Source: three-view drawing plus pictorial views. Frame: mm from the lowest corner of the part. Coordinates: 2 decimals unless noted, no trailing zeros. Order: outer loops, then holes, each group sorted by start corner. A loop starts at its lowest first (then second) coordinate and runs counter-clockwise, first axis right, second up. Notation, with made-up numbers: M -28,17 L 12,17 A24 cw 12,33 Z; hole C 38,-19.5 d11. An arc over 180 degrees is marked long. Use CSV: the item, a comma, the result in double quotes. Start each with the question number.
Q1. Section query B-B, the plane y = 7.25. Output: boundary loops of the cut face in (x, z), and give its area (3 significant figures).
Q2. Section query C-C, the plane z = 64. Output: boundary loops of the cut face in (x, y), and give its area (3 significant figures).
Q3. First-contact query: P1, Ø2.5, axis at y = 8, z = 28, coming from the +X side; P2, Ø3, axis at x = 1.5, y = 4, coming from the -Z side; P3, Ø1, axis at x = 2.5, z = 42, coming from the +Y side. Flat tips, straight axial feed; report the tip coordinate or a pass-through.
Q4. Section query D-D, the plane x = 4. Output: boundary loops of the cut face in (y, z), and give its area (3 significant figures).
Q5. Ray query, probe 1 along X at (y, z) = (2, 89.5); probe 2 along X at (y, z) = (4.75, 79); probe 3 along Z at (x, y) = (5.75, 1). Return the intervals inside material, ascending.
Q6. Section query A-A, the plane z = 8. Output: boundary loops of the cut face in (x, y).
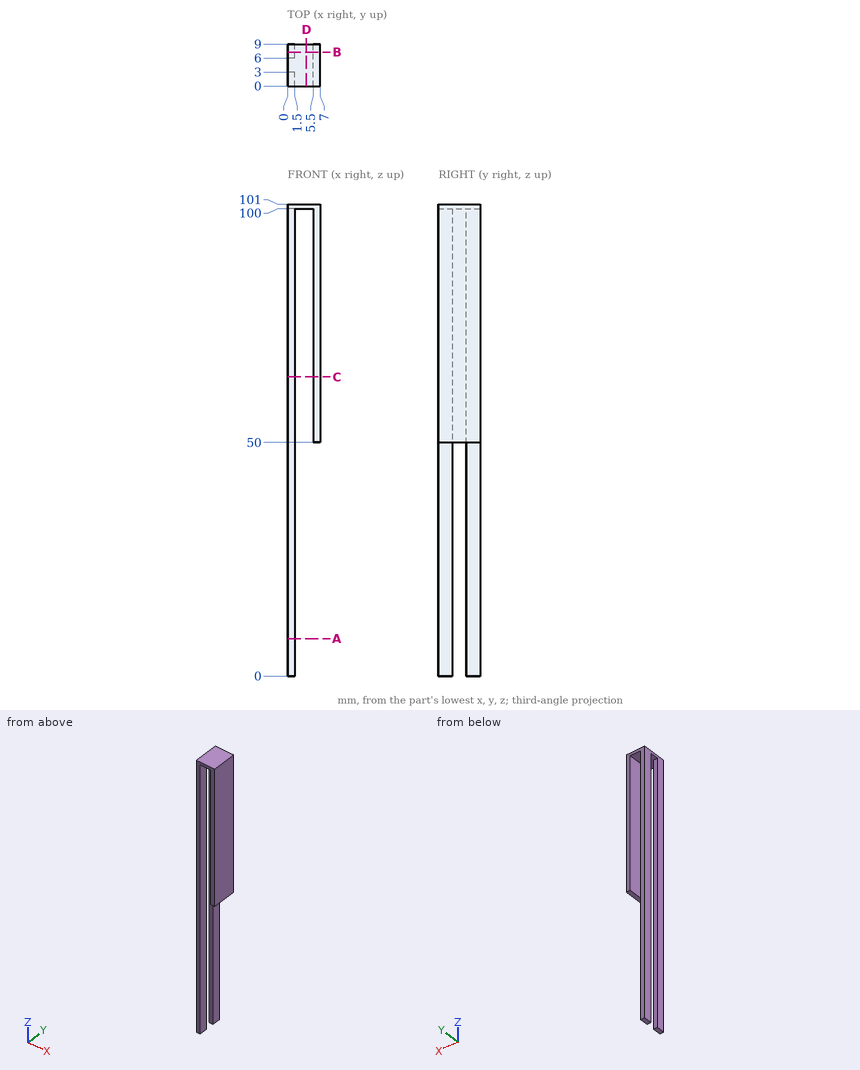
Responses:
1,outline,"M 0,0 L 1.5,0 L 1.5,100 L 5.5,100 L 5.5,50 L 7,50 L 7,101 L 0,101 Z"
1,area,"232 mm²"
2,outline,"M 0,0 L 1.5,0 L 1.5,3 L 0,3 Z; M 0,6 L 1.5,6 L 1.5,9 L 0,9 Z; M 5.5,0 L 7,0 L 7,9 L 5.5,9 Z"
2,area,"22.5 mm²"
3,P1,"stops at x = 1.5"
3,P2,"stops at z = 0"
3,P3,"passes through"
4,outline,"M 0,100 L 9,100 L 9,101 L 0,101 Z"
4,area,"9.00 mm²"
5,probe 1,"x = 0 to 1.5, 5.5 to 7"
5,probe 2,"x = 5.5 to 7"
5,probe 3,"z = 50 to 101"
6,outline,"M 0,0 L 1.5,0 L 1.5,3 L 0,3 Z; M 0,6 L 1.5,6 L 1.5,9 L 0,9 Z"
